The listing builds one solid part. Answer for the finished solid, in the listing's coordinates (mm). A direction names the side the tool comes from. Give positions to 0.01 mm unless a question says otherwise; leave off trailing zeros. Order: outer loops, then holes, each group sorted by start corner. A loop starts at its lowest first (then second) coordinate and runs counter-clockwise, first axis right, second up. Notation, with made-up numbers: (53.25, 17) - (62.25, 17) arc R22 cw to (62.25, 36) - close; hole circle Ø2 at (-31.5, -38). An arc over 180 degrees is marked (long way). Answer in a Markdown table with one row per item. Add a question column.
```python
from build123d import *

# Parameters (mm, degrees)
Y_KSEKLIK_EKSTR_ZYON1_DEPTH = 5
IZIM6_W                     = 83
IZIM6_H                     = 46
KES_EKSTR_ZYON2_DEPTH       = 4
RADYUS1_R                   = 4
IZIM7_R                     = 1
KES_EKSTR_ZYON3_DEPTH       = 1000
IZIM9_R                     = 1.75
KES_EKSTR_ZYON5_DEPTH       = 1
KES_EKSTR_ZYON6_START       = -1
IZIM10_R                    = 1.75
KES_EKSTR_ZYON6_DEPTH       = 1


with BuildPart() as part:
    # Çizim4 → Yükseklik-Ekstrüzyon1 (new body)
    with BuildSketch(Plane.XY):
        with BuildLine():
            Line((202.815557626, -67.077395959), (202.815557626, -82.077395959))
            ThreePointArc((202.815557626, -82.077395959), (192.815557626, -92.077395959), (202.815557626, -102.077395959))
            Line((202.815557626, -102.077395959), (202.815557626, -117.077395959))
            Line((202.815557626, -117.077395959), (202.815557626, -120.077395959))
            Line((202.815557626, -120.077395959), (179.315557626, -120.077395959))
            Line((179.315557626, -120.077395959), (179.315557626, -119.077395959))
            ThreePointArc((179.315557626, -119.077395959), (177.551625603, -117.605260004), (175.315557626, -117.077395959))
            Line((175.315557626, -117.077395959), (143.315557626, -117.077395959))
            ThreePointArc((143.315557626, -117.077395959), (141.079489648, -117.605260004), (139.315557626, -119.077395959))
            Line((139.315557626, -119.077395959), (139.315557626, -120.077395959))
            Line((139.315557626, -120.077395959), (114.815557626, -120.077395959))
            Line((114.815557626, -120.077395959), (114.815557626, -104.577395959))
            Line((114.815557626, -104.577395959), (115.815557626, -104.577395959))
            ThreePointArc((115.815557626, -104.577395959), (117.287693581, -102.813463937), (117.815557626, -100.577395959))
            Line((117.815557626, -100.577395959), (117.815557626, -83.577395959))
            ThreePointArc((117.815557626, -83.577395959), (117.287693581, -81.341327982), (115.815557626, -79.577395959))
            Line((115.815557626, -79.577395959), (114.815557626, -79.577395959))
            Line((114.815557626, -79.577395959), (114.815557626, -64.077395959))
            Line((114.815557626, -64.077395959), (139.315557626, -64.077395959))
            Line((139.315557626, -64.077395959), (139.315557626, -65.077395959))
            ThreePointArc((139.315557626, -65.077395959), (141.079489648, -66.549531914), (143.315557626, -67.077395959))
            Line((143.315557626, -67.077395959), (175.315557626, -67.077395959))
            ThreePointArc((175.315557626, -67.077395959), (177.551625603, -66.549531914), (179.315557626, -65.077395959))
            Line((179.315557626, -65.077395959), (179.315557626, -64.077395959))
            Line((179.315557626, -64.077395959), (202.815557626, -64.077395959))
            Line((202.815557626, -64.077395959), (202.815557626, -67.077395959))
        make_face()
    extrude(amount=Y_KSEKLIK_EKSTR_ZYON1_DEPTH)

    # Çizim6 → Kes-Ekstrüzyon2 (cut)
    with BuildSketch(Plane.XY.offset(5)):
        with Locations((161.315557626, -92.077395959)):
            Rectangle(IZIM6_W, IZIM6_H)
    extrude(amount=-KES_EKSTR_ZYON2_DEPTH, mode=Mode.SUBTRACT)

    # Radyus1
    # the kernel refuses this fillet: 4 mm, written as the material it takes off along each edge
    with BuildSketch(Plane(origin=(155.315557626, -64.077395959, 0), x_dir=(0, -1, 0), z_dir=(1, 0, 0)), Plane(origin=(226.815557626, -120.077395959, 0), x_dir=(0, 1, 0), z_dir=(-1, 0, 0))) as radyus1_piece_1:
        with BuildLine():
            CenterArc((RADYUS1_R, -RADYUS1_R), RADYUS1_R, 90, 90)
            Line((0, -RADYUS1_R), (-RADYUS1_R * 0.02, -RADYUS1_R))
            Line((-RADYUS1_R * 0.02, -RADYUS1_R), (-RADYUS1_R * 0.02, RADYUS1_R * 0.02))
            Line((-RADYUS1_R * 0.02, RADYUS1_R * 0.02), (RADYUS1_R, RADYUS1_R * 0.02))
            Line((RADYUS1_R, RADYUS1_R * 0.02), (RADYUS1_R, 0))
        make_face()
    extrude(amount=71.5, mode=Mode.SUBTRACT)
    with BuildSketch(Plane(origin=(163.315557626, -120.077395959, 0), x_dir=(0, 1, 0), z_dir=(-1, 0, 0)), Plane(origin=(90.815557626, -64.077395959, 0), x_dir=(0, -1, 0), z_dir=(1, 0, 0))) as radyus1_piece_2:
        with BuildLine():
            CenterArc((RADYUS1_R, -RADYUS1_R), RADYUS1_R, 90, 90)
            Line((0, -RADYUS1_R), (-RADYUS1_R * 0.02, -RADYUS1_R))
            Line((-RADYUS1_R * 0.02, -RADYUS1_R), (-RADYUS1_R * 0.02, RADYUS1_R * 0.02))
            Line((-RADYUS1_R * 0.02, RADYUS1_R * 0.02), (RADYUS1_R, RADYUS1_R * 0.02))
            Line((RADYUS1_R, RADYUS1_R * 0.02), (RADYUS1_R, 0))
        make_face()
    extrude(amount=72.5, mode=Mode.SUBTRACT)
    with BuildSketch(Plane(origin=(114.815557626, -144.077395959, 0), x_dir=(1, 0, 0), z_dir=(0, 1, 0)), Plane(origin=(114.815557626, -103.577395959, 0), x_dir=(1, 0, 0), z_dir=(0, 1, 0))) as radyus1_piece_3:
        with BuildLine():
            CenterArc((RADYUS1_R, -RADYUS1_R), RADYUS1_R, 90, 90)
            Line((0, -RADYUS1_R), (-RADYUS1_R * 0.02, -RADYUS1_R))
            Line((-RADYUS1_R * 0.02, -RADYUS1_R), (-RADYUS1_R * 0.02, RADYUS1_R * 0.02))
            Line((-RADYUS1_R * 0.02, RADYUS1_R * 0.02), (RADYUS1_R, RADYUS1_R * 0.02))
            Line((RADYUS1_R, RADYUS1_R * 0.02), (RADYUS1_R, 0))
        make_face()
    extrude(amount=63.5, mode=Mode.SUBTRACT)

    # Çizim7 → Kes-Ekstrüzyon3 (cut)
    with BuildSketch(Plane(origin=(0, -67.077395959, 0), x_dir=(1, 0, 0), z_dir=(0, 1, 0))):
        with Locations(Location((159.315557626, -3, 0), (0, 0, 270))):
            Circle(IZIM7_R)
    extrude(amount=-KES_EKSTR_ZYON3_DEPTH, mode=Mode.SUBTRACT)

    # Çizim9 → Kes-Ekstrüzyon5 (cut)
    with BuildSketch(Plane(origin=(0, -117.077395959, 0), x_dir=(-1, 0, 0), z_dir=(0, -1, 0))):
        with Locations(Location((-159.315557626, -3, 0), (0, 0, 90))):
            Circle(IZIM9_R)
    extrude(amount=-KES_EKSTR_ZYON5_DEPTH, mode=Mode.SUBTRACT)

    # Çizim10 → Kes-Ekstrüzyon6 (cut)
    with BuildSketch(Plane(origin=(0, -67.077395959, 0), x_dir=(1, 0, 0), z_dir=(0, 1, 0)).offset(KES_EKSTR_ZYON6_START)):
        with Locations(Location((159.315557626, -3, 0), (0, 0, 90))):
            Circle(IZIM10_R)
    extrude(amount=KES_EKSTR_ZYON6_DEPTH, mode=Mode.SUBTRACT)


solid = part.part
```
(1) Find section C-C, the plane z = 3. Give the number of separate pieces and of enclosed holes in the cut face, plus the area to 3 significant figures.
(2) Find section D-D, the plane x = 173. Write down the section's boundary in (y, z), plus the area to 3 significant figures.
(3) The mould has two halves that part along X. Classify faces 5 (the face through (159, -67.077, 1)), 6 (the face through (117.3, -81.37, 2.53)), 7 (the face through (159.43, -116.38, 0.01)): +X half, -X half, draft (parallel to the pull), parting line (faces both ways), or undercut.
(4) Straight lines are drawn through the part: line 1 (Y direction, x = 179.5, z = 4); line 2 (Y direction, x = 172, z = 4.35); line 3 (Z direction, x = 186, y = -87). For each, find the intervals that lie inside material, in ascending order.
(5) For faces 1 (the face through (161, -115.077, 3)), 2 (the face through (161.05, -116.58, 3.23)), 3 (the face through (117.273, -102.842, 2.529)), 4 (the face through (141.11, -117.59, 2.53)), determine the directions among +Z, -Z, +X, -X, +Y, -Y from which every point of the face is accessible in a straight line to the end or side of a thin tool.
(6) Find section A-A, the plane x = 190. Write down the section's boundary in (y, z), plus the area to 3 significant figures.
(7) Each of these flat-tipped pins is pushed along its axis until it touches: P1, Ø1, axis at x = 159.5, z = 3.5, coming from the -Y side; P2, Ø14, axis at x = 161.5, y = -89, coming from the +Z side; P3, Ø1.5, axis at x = 157, z = 2.5, coming from the -Y side. Where does it stop, or does it pass through?
(8) Find section B-B, the plane y = -73. Write down the section's boundary in (x, z).
Answer key:
| question | item | result |
|---|---|---|
| 1 | separate pieces | 3 |
| 1 | enclosed holes | 0 |
| 1 | area | 782 mm² |
| 2 | outline | (-117.08, 0.13) arc R4 ccw to (-116.08, 0) - (-68.08, 0) arc R4 ccw to (-67.08, 0.13) - (-67.08, 5) - (-69.08, 5) - (-69.08, 1) - (-115.08, 1) - (-115.08, 5) - (-117.08, 5) - close |
| 2 | area | 65.9 mm² |
| 3 | face 5 | undercut |
| 3 | face 6 | -X half |
| 3 | face 7 | draft |
| 4 | line 1 | -120.08 to -115.08, -69.08 to -64.08 |
| 4 | line 2 | -117.08 to -115.08, -69.08 to -67.08 |
| 4 | line 3 | 0 to 1 |
| 5 | face 1 | +Z, +X |
| 5 | face 2 | -Y |
| 5 | face 3 | +Z, -Z, -X |
| 5 | face 4 | +Z, -Z, -Y |
| 6 | outline | (-120.08, 4) arc R4 ccw to (-116.08, 0) - (-68.08, 0) arc R4 ccw to (-64.08, 4) - (-64.08, 5) - (-69.08, 5) - (-69.08, 1) - (-115.08, 1) - (-115.08, 5) - (-120.08, 5) - close |
| 6 | area | 89.1 mm² |
| 7 | P1 | y = -116.08 |
| 7 | P2 | z = 1 |
| 7 | P3 | y = -117.08 |
| 8 | outline | (114.82, 4) arc R4 ccw to (118.82, 0) - (202.82, 0) - (202.82, 1) - (119.82, 1) - (119.82, 5) - (114.82, 5) - close |
